Autodesk Fusion 360 part; units mm, degrees
sketch "Sketch1" plane through (0, 0, 0) normal (0, 0, 1) x (1, 0, 0)
  arc A0 (31.75, 63.5) -> (-31.75, 63.5) centre (0, 63.5) ccw
  arc A1 (-31.75, 0) -> (31.75, 0) centre (0, 0) ccw
  line L0 (0, 0) -> (0, 63.5) construction
  circle A2 centre (0, 63.5) radius 14.2748
  circle A3 centre (0, 0) radius 14.2748
  arc A4 (-31.75, 37.5429) -> (-31.75, 24.8429) centre (-31.75, 31.1929) ccw
  arc A5 (31.75, 24.8429) -> (31.75, 37.5429) centre (31.75, 31.1929) ccw
  line L1 (-31.75, 63.5) -> (-31.75, 37.5429)
  line L2 (-31.75, 24.8429) -> (-31.75, 0)
  line L3 (31.75, 0) -> (31.75, 24.8429)
  line L4 (31.75, 37.5429) -> (31.75, 63.5)
  circle A6 centre (0, 0) radius 31.75 construction
  circle A7 centre (0, 63.5) radius 31.75 construction
  circle A8 centre (31.75, 31.1929) radius 2.5797
  circle A9 centre (-31.75, 31.1929) radius 2.5797
  dimension "d1" = 63.5
  dimension "d2" = 28.5496
  dimension "d3" = 28.5496
  dimension "d4" = 63.5
  dimension "d5" = 12.7
  dimension "d6" = 12.7
  dimension "d7" = 63.5
  dimension "d8" = 63.5
  dimension "d9" = 5.1594
  dimension "d10" = 5.1594
extrude "Extrude1" add sketch "Sketch1" along normal blind 6.35
equation "d9 = ( 13 / 64 ) * 1 in"
equation "d10 = ( 13 / 64 ) * 1 in"
For this review, take the finished solid that the model builds, in its own axes (mm). A direction names the side the tool comes from. Coordinates: 2 decimals unless noted, no trailing zeros. Loops run counter-clockwise (first coordinate to the right, second up) from the corner with the lowest first, then second, coordinate; pieces in that order, holes last. Notation, with made-up numbers: (-0.75, -0.75) - (31.25, -0.75) arc R24 ccw to (31.25, 37.25) - close; hole circle Ø2 at (45.25, 48.25). An arc over 180 degrees is marked (long way). Return JSON: item names as keys, results as strings.
Item 1: Take a section at A-A (x = 0). Give the boundary of the cut face in (y, z), then the cut area to 3 significant figures.
Determined:
{"outline": "(-31.75, 0) - (-14.27, 0) - (-14.27, 6.35) - (-31.75, 6.35) - close; (14.27, 0) - (49.23, 0) - (49.23, 6.35) - (14.27, 6.35) - close; (77.77, 0) - (95.25, 0) - (95.25, 6.35) - (77.77, 6.35) - close", "area": "444 mm2"}
Item 2: Take a section at C-C (z = 1.75). Give the boundary of the cut face in (x, y), then the cut area to 3 significant figures.
Determined:
{"outline": "(-31.75, 0) arc R31.75 ccw to (31.75, 0) - (31.75, 24.84) arc R6.35 ccw to (31.75, 37.54) - (31.75, 63.5) arc R31.75 ccw to (-31.75, 63.5) - (-31.75, 37.54) arc R6.35 ccw to (-31.75, 24.84) - close; hole circle Ø5.16 at (-31.75, 31.19); hole circle Ø28.55 at (0, 0); hole circle Ø28.55 at (0, 63.5); hole circle Ø5.16 at (31.75, 31.19)", "area": "6,000 mm2"}
Item 3: For faces 1 (the flat face through (-31.75, 13, 3)), 2 (the flat face through (-31.75, 51, 3)), 3 (the flat face through (31.75, 50, 3)), list the 3-axis set-ups (+Z, -Z, +X, -X, +Y, -Y) from which the entire face can be reached by the end or side of a thin tool; tool diameter is ignored.
Determined:
{"face 1": "+Z, -Z, -X, -Y", "face 2": "+Z, -Z, -X, +Y", "face 3": "+Z, -Z, +X, +Y"}
Item 4: Mouldability with a two-part tool opening along Y and no side actions: class faces 4 (the cylindrical face through (-14.26, -0.63, 3.13)), 5 (the flat face through (31.75, 12, 3)), 6 (the cylindrical face through (-0.698, 95.242, 3.131)), 7 (the cylindrical face through (31.19, 33.71, 3.13)) as pulls with the +Y half, pulls with the -Y half, needs draft (parallel to the pull), parting line crosses it, or undercut.
Determined:
{"face 4": "undercut", "face 5": "needs draft", "face 6": "pulls with the +Y half", "face 7": "undercut"}
Item 5: Take a section at B-B (y = 66.5). Give the boundary of the cut face in (x, z).
Determined:
{"outline": "(-31.61, 0) - (-13.96, 0) - (-13.96, 6.35) - (-31.61, 6.35) - close; (13.96, 0) - (31.61, 0) - (31.61, 6.35) - (13.96, 6.35) - close"}
Item 6: Take a section at D-D (x = 24.5). Give the boundary of the cut face in (y, z), then the cut area to 3 significant figures.
Determined:
{"outline": "(-20.19, 0) - (83.69, 0) - (83.69, 6.35) - (-20.19, 6.35) - close", "area": "660 mm2"}
Item 7: For line 1 (Y direction, x = 0, z = 3.5); line 2 (Y direction, x = 7.5, z = 2); line 3 (X direction, y = -8, z = 1.5), list the stretches that pass through material, from the lowest coordinate up.
Determined:
{"line 1": "y = -31.75 to -14.27, 14.27 to 49.23, 77.77 to 95.25", "line 2": "y = -30.85 to -12.15, 12.15 to 51.35, 75.65 to 94.35", "line 3": "x = -30.73 to -11.82, 11.82 to 30.73"}
Item 8: Insertion check: pin 1 (3 mm diameter, centred on y = 46.5, z = 2.5, fed in from -X); pin 2 (1.9 mm diameter, centred on y = 15, z = 3, fed in from +X); pin 3 (4 mm diameter, centred on x = 31.75, y = 31.19, fed in from +Z). Each pin has a flat end and moves straight along its axis. Give the tip position at first contact, or say it passes through.
Determined:
{"pin 1": "stops at x = -31.75", "pin 2": "stops at x = 31.75", "pin 3": "passes through"}
